from build123d import *

# Parameters (mm, degrees)
SKETCH1_R           = 76.2
BOSS_EXTRUDE1_DEPTH = 28.575
SKETCH2_R           = 9.525
CUT_EXTRUDE1_DEPTH  = 112.48726665
SKETCH30_R          = 3.175
CUT_EXTRUDE2_DEPTH  = 25.4
CIRPATTERN3_COUNT   = 4
SKETCH31_R          = 6.35
CUT_EXTRUDE3_DEPTH  = 112.487266812
CIRPATTERN4_COUNT   = 4
SKETCH34_W          = 2.54
SKETCH34_H          = 14.2875


with BuildPart() as part:
    # Sketch1 → Boss-Extrude1 (new body)
    with BuildSketch(Plane(origin=(0, 0, 0), x_dir=(1, 0, 0), z_dir=(0, 1, 0))):
        with Locations(Location((0, 0, 0), (0, 0, 270))):
            Circle(SKETCH1_R)
    extrude(amount=BOSS_EXTRUDE1_DEPTH)

    # Sketch2 → Cut-Extrude1 (cut, through all)
    with BuildSketch(Plane(origin=(0, 28.575, 0), x_dir=(1, 0, 0), z_dir=(0, 1, 0))):
        with Locations(Location((0, 0, 0), (0, 0, 270))):
            Circle(SKETCH2_R)
    extrude(amount=-CUT_EXTRUDE1_DEPTH, mode=Mode.SUBTRACT)

    # Sketch30 → Cut-Extrude2 (cut)
    with BuildSketch(Plane.XY.offset(76.2)):
        with Locations((0, 22.225)):
            Circle(SKETCH30_R)
        with Locations((0, 6.35)):
            Circle(SKETCH30_R)
    cut_extrude2 = extrude(amount=-CUT_EXTRUDE2_DEPTH, mode=Mode.SUBTRACT)

    # CirPattern3: Cut-Extrude2 ×4 about axis
    cirpattern3_axis = Axis((0, 0, 0), (0, 1, 0))
    for i in range(1, CIRPATTERN3_COUNT):
        add(cut_extrude2.rotate(cirpattern3_axis, i * 360 / CIRPATTERN3_COUNT), mode=Mode.SUBTRACT)

    # Sketch31 → Cut-Extrude3 (cut, through all)
    with BuildSketch(Plane(origin=(0, 28.575, 0), x_dir=(1, 0, 0), z_dir=(0, 1, 0))):
        with Locations(Location((35.921024484, 35.921024484, 0), (0, 0, 270))):
            Circle(SKETCH31_R)
    cut_extrude3 = extrude(amount=-CUT_EXTRUDE3_DEPTH, mode=Mode.SUBTRACT)

    # CirPattern4: Cut-Extrude3 ×4 about axis
    cirpattern4_axis = Axis((0, 0, 0), (0, 1, 0))
    for i in range(1, CIRPATTERN4_COUNT):
        add(cut_extrude3.rotate(cirpattern4_axis, i * 360 / CIRPATTERN4_COUNT), mode=Mode.SUBTRACT)

    # Sketch34 → Cut-Revolve1 (revolve, cut)
    with BuildSketch(Plane.XY, mode=Mode.PRIVATE) as cut_revolve1_sk:
        with Locations((74.93, 21.43125)):
            Rectangle(SKETCH34_W, SKETCH34_H)
    revolve(cut_revolve1_sk.sketch.rotate(Axis((0, 28.575, 0), (0, -1, 0)), 90), axis=Axis((0, 28.575, 0), (0, -1, 0)), mode=Mode.SUBTRACT)


solid = part.part
Read the model definition and answer for the solid it produces. Units are mm, in the model's axes. A direction names the side the tool comes from. Round coordinates to 2 decimals unless told otherwise and drop trailing zeros. Write each loop counter-clockwise with the first axis right and the second up, starting at its lowest first coordinate (ties: lowest second). Pieces come first, ordered by that corner, then holes.
Q1. Find section D-D on y = 6.35. Determine the outline of the cut face in (x, z) (3 decimals), and give its area (3 significant figures).
Values:
outline: (-76.134, -3.175) arc R76.2 ccw to (-3.175, -76.134) - (-3.175, -50.8) - (3.175, -50.8) - (3.175, -76.134) arc R76.2 ccw to (76.134, -3.175) - (50.8, -3.175) - (50.8, 3.175) - (76.134, 3.175) arc R76.2 ccw to (3.175, 76.134) - (3.175, 50.8) - (-3.175, 50.8) - (-3.175, 76.134) arc R76.2 ccw to (-76.134, 3.175) - (-50.8, 3.175) - (-50.8, -3.175) - close; hole circle Ø12.7 at (-35.921, -35.921); hole circle Ø12.7 at (-35.921, 35.921); hole circle Ø19.05 at (0, 0); hole circle Ø12.7 at (35.921, -35.921); hole circle Ø12.7 at (35.921, 35.921)
area: 16,800 mm2
Q2. The mould has two halves that part along X. Classify faces 1 (the face through (0.413, 25.373, -62.391)), 2 (the face through (-22.125, 21.531, 70.259)), 3 (the face through (-62.391, 25.373, -0.413)): released by +X, released by -X, zero draft, split by the parting line, or undercut.
Values:
face 1: undercut
face 2: split by the parting line
face 3: zero draft
Q3. Find section C-C on z = -40.5. Determine the outline of the cut face in (x, y) (1 decimal).
Values:
outline: (-64.5, 0) - (-40.3, 0) - (-40.3, 28.6) - (-61.5, 28.6) - (-61.5, 14.3) - (-64.5, 14.3) - close; (-31.5, 0) - (31.5, 0) - (31.5, 28.6) - (-31.5, 28.6) - close; (40.3, 0) - (64.5, 0) - (64.5, 14.3) - (61.5, 14.3) - (61.5, 28.6) - (40.3, 28.6) - close
Q4. Flat-ended cylindrical pins translate along their axes: P1, Ø5, axis at x = 41, y = 24, coming from the +Z side; P2, Ø1.5, axis at x = 37.5, y = 7, coming from the +Z side; P3, Ø10, axis at x = 0, y = 22.225, coming from the +Z side. Find the tip coordinate at first contact, or state that the pin passes through.
Values:
P1: stops at z = 62.8
P2: stops at z = 66.75
P3: stops at z = 73.66
Q5. A tool of negligible diameter and unlimited length cuts with its end or side. For faces 4 (the face through (0, 6, 50.8)), 5 (the face through (50.8, 22, 0)), 6 (the face through (-42.265, 14.488, -36.2)), 7 (the face through (-1.707, 9.027, -63.678)), from which of +Z, -Z, +X, -X, +Y, -Y can it reach the whole face along a straight path? Write none if from no direction.
Values:
face 4: +Z
face 5: +X
face 6: +Y, -Y
face 7: -Z
Q6. Straight lines are drawn through the part: line 1 (Y direction, x = -68, z = 0) (3 decimals); line 2 (X direction, y = 27.25, z = -31); line 3 (Z direction, x = -68, y = 8.5). For each, find the intervals that lie inside material, in ascending order.
Values:
line 1: y = 0 to 3.175, 9.525 to 19.05, 25.4 to 28.575
line 2: x = -66.82 to -39.93, -31.91 to 31.91, 39.93 to 66.82
line 3: z = -34.39 to -2.34, 2.34 to 34.39
